CAD build for the part. Positions are in the model's coordinates, mm. Face numbers are marked on the shaded views. A direction names the side the tool comes from. Round coordinates to 2 decimals unless told otherwise and drop trailing zeros. Order: outer loops, then holes, each group sorted by start corner. A loop starts at its lowest first (then second) coordinate and runs counter-clockwise, first axis right, second up. Notation, with made-up numbers: M 27,88 L 32,88 A12 ccw 32,109 Z; hole C -5.75,87.25 d1. An arc over 180 degrees is marked long. Put each result on its own line as item: value.
```python
from build123d import *

# Parameters (mm, degrees)
SKETCH_1_R         = 4
EXTRUDE_1_DEPTH    = 58
HOLE_WIZARD_M4_1_D = 3.3


with BuildPart() as part:
    # 草图1 → 凸台-拉伸1 (new body)
    with BuildSketch(Plane.XY):
        Polygon((8.5, 0), (-8.5, 0), (-8.5, 1.5), (-11, 4), (-17, 4), (-17, 22), (17, 22), (17, 4), (11, 4), (8.5, 1.5), align=None)
        with Locations(Location((0, 11, 0), (0, 0, 180))):
            Circle(SKETCH_1_R, mode=Mode.SUBTRACT)
    extrude(amount=EXTRUDE_1_DEPTH)

    # M4 螺纹孔1 (through all)
    with Locations(Plane(origin=(0, 22, 0), x_dir=(-1, 0, 0), z_dir=(0, 1, 0))):
        with Locations((12, 50), (-12, 50), (-12, 8), (12, 8)):
            Hole(HOLE_WIZARD_M4_1_D / 2)


solid = part.part
```
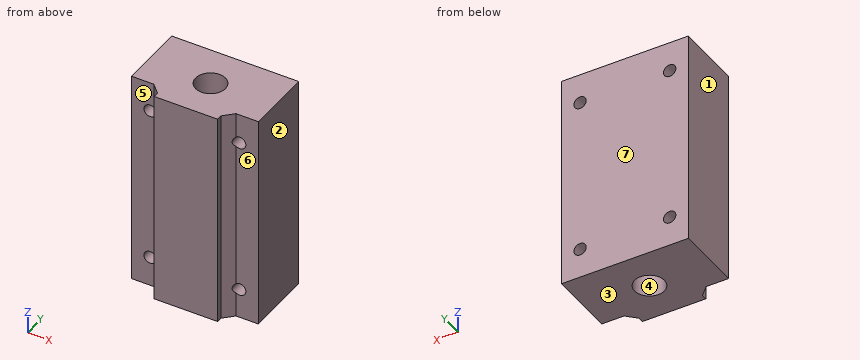
Item 1: Band-saw the part on A-A on z = 50. Give the cut face in (x, y), and give its area (3 significant figures).
Answers below:
outline: M -17,4 L -13.65,4 L -13.65,22 L -17,22 Z; M -10.35,3.35 L -8.5,1.5 L -8.5,0 L 8.5,0 L 8.5,1.5 L 10.35,3.35 L 10.35,22 L -10.35,22 Z; M 13.65,4 L 17,4 L 17,22 L 13.65,22 Z; hole C 0,11 d8
area: 517 mm²
Item 2: Tool access for the marked faces 5, 6 and 7: list every direction of +Z, -Z, +X, -X, +Y, -Y with a clear straight run to the whole face (end or side of a thin tool).
Answers below:
face 5: +Z, -Z, -X, -Y
face 6: +Z, -Z, +X, -Y
face 7: +Z, -Z, +X, -X, +Y
Item 3: Probe line 1 along Z through (x, y) = (12, 7.25); line 2 along X through (y, z) = (15.5, 8); line 3 along X through (y, z) = (14, 50). List the from-to ranges inside material, lowest first. Write a range as [from, to].
Answers below:
line 1: [0, 6.35], [9.65, 48.35], [51.65, 58]
line 2: [-17, -13.65], [-10.35, 10.35], [13.65, 17]
line 3: [-17, -13.65], [-10.35, -2.65], [2.65, 10.35], [13.65, 17]
Item 4: Band-saw the part on C-C on y = 11. Give the cut face in (x, z), and give its area (3 significant figures).
Answers below:
outline: M -17,0 L -4,0 L -4,58 L -17,58 Z; M 4,0 L 17,0 L 17,58 L 4,58 Z; hole C -12,8 d3.3; hole C -12,50 d3.3; hole C 12,8 d3.3; hole C 12,50 d3.3
area: 1,470 mm²
Item 5: Band-saw the part on D-D on x = -12. Give the cut face in (y, z), and give its area (3 significant figures).
Answers below:
outline: M 4,0 L 22,0 L 22,6.35 L 4,6.35 Z; M 4,9.65 L 22,9.65 L 22,48.35 L 4,48.35 Z; M 4,51.65 L 22,51.65 L 22,58 L 4,58 Z
area: 925 mm²
Item 6: Pin check, flat tips, straight feed: P1, Ø3, axis at x = 13.5, z = 24, coming from the -Y side; P2, Ø1.2, axis at y = 0.5, z = 31, coming from the -X side; P3, Ø4, axis at x = 12, z = 38.5, coming from the -Y side. Stop position of each tip, or through.
Answers below:
P1: y = 4
P2: x = -8.5
P3: y = 3
Item 7: Band-saw the part on B-B on x = 0. Give the cut face in (y, z), and give its area (3 significant figures).
Answers below:
outline: M 0,0 L 7,0 L 7,58 L 0,58 Z; M 15,0 L 22,0 L 22,58 L 15,58 Z
area: 812 mm²
Item 8: Mould opens along X. For the marked faces 1, 2, 3 and 4 say: pulls with the +X half, pulls with the -X half, needs draft (parallel to the pull), parting line crosses it, or undercut.
Answers below:
face 1: pulls with the -X half
face 2: pulls with the +X half
face 3: needs draft
face 4: undercut
